Can you work these out from the model? Positions are in its coordinate system, mm. Give positions to 0.01 mm unless a question says otherwise; leave off trailing zeros. Order: outer loops, then holes, each group sorted by start corner. A loop starts at its lowest first (then second) coordinate and runs counter-clockwise, first axis right, second up. Notation, with made-up numbers: (63, 48.5) - (111, 48.5) arc R21 cw to (111, 62.5) - close; hole circle Ø7 at (-30, 39.5). An arc over 180 degrees is marked (long way). Answer as a JSON object with one key per item and string values.
```python
from build123d import *

# Parameters (mm, degrees)
SKETCH3_W               = 70
SKETCH3_H               = 70
BOSS_EXTRUDE2_DEPTH     = 1.31
CUT_EXTRUDE1_DEPTH      = 3.08
CUT_EXTRUDE1_DEPTH_BACK = 31
SKETCH4_R               = 3
SKETCH4_W               = 30
SKETCH4_H               = 30


with BuildPart() as part:
    # Sketch3 → Boss-Extrude2 (new body)
    with BuildSketch(Plane.XY):
        Rectangle(SKETCH3_W, SKETCH3_H)
    extrude(amount=BOSS_EXTRUDE2_DEPTH)

    # Sketch4 → Cut-Extrude1 (cut, two sides: drawn at the far end of the back side and taken through both)
    with BuildSketch(Plane.XY.offset(1.31).offset(-CUT_EXTRUDE1_DEPTH_BACK)):
        with Locations(Location((-25, 25, 0), (0, 0, 180))):
            Circle(SKETCH4_R)
        with Locations(Location((0, 25, 0), (0, 0, 180))):
            Circle(SKETCH4_R)
        with Locations(Location((25, 25, 0), (0, 0, 180))):
            Circle(SKETCH4_R)
        with Locations(Location((25, 0, 0), (0, 0, 180))):
            Circle(SKETCH4_R)
        with Locations(Location((25, -25, 0), (0, 0, 180))):
            Circle(SKETCH4_R)
        with Locations(Location((0, -25, 0), (0, 0, 180))):
            Circle(SKETCH4_R)
        with Locations(Location((-25, -25, 0), (0, 0, 180))):
            Circle(SKETCH4_R)
        with Locations(Location((-25, 0, 0), (0, 0, 180))):
            Circle(SKETCH4_R)
        Rectangle(SKETCH4_W, SKETCH4_H)
    extrude(amount=CUT_EXTRUDE1_DEPTH + CUT_EXTRUDE1_DEPTH_BACK, mode=Mode.SUBTRACT)


solid = part.part
```
Q1. If we section it at D-D, the plane y = 25: Please give me the cut outline in (x, z).
Recorded:
{"outline": "(-35, 0) - (-28, 0) - (-28, 1.31) - (-35, 1.31) - close; (-22, 0) - (-3, 0) - (-3, 1.31) - (-22, 1.31) - close; (3, 0) - (22, 0) - (22, 1.31) - (3, 1.31) - close; (28, 0) - (35, 0) - (35, 1.31) - (28, 1.31) - close"}
Q2. If we section it at A-A, the plane y = 4: Please give me the cut outline in (x, z).
Recorded:
{"outline": "(-35, 0) - (-15, 0) - (-15, 1.31) - (-35, 1.31) - close; (15, 0) - (35, 0) - (35, 1.31) - (15, 1.31) - close"}
Q3. I'm going to push a flat-ended pin straight in: pin 1 Ø5 at (x, y) = (25, 25) entering from -Z. Where does the tip first touch, or does it pass through?
Recorded:
{"pin 1": "passes through"}
Q4. If we section it at C-C, the plane z = 0.2: Count the separate pieces of the cut face and the enclosed holes in it, then the cut area to 3 significant figures.
Recorded:
{"separate pieces": "1", "enclosed holes": "9", "area": "3,770 mm^2"}
Q5. I need wall thicknesses on L1, parallel to Y at x = 25, z = 0.55; L2, parallel to Y at x = 5.5, z = 0.45. Which ranges of each line are inside material? Lowest first, please.
Recorded:
{"L1": "y = -35 to -28, -22 to -3, 3 to 22, 28 to 35", "L2": "y = -35 to -15, 15 to 35"}
Q6. We'd pull the mould along Y, two halves only. Please class faces 1 (the face through (0, 16, 1.31)), 2 (the face through (28, 0, 1)): released by +Y, released by -Y, zero draft, split by the parting line, or undercut.
Recorded:
{"face 1": "zero draft", "face 2": "undercut"}
